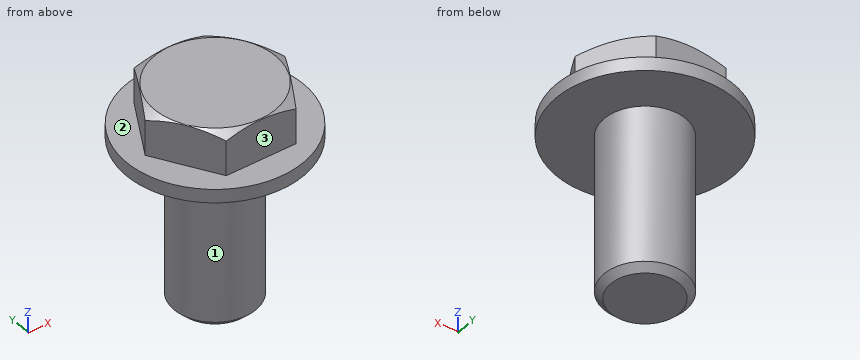
Solid Edge part; units mm, degrees
sketch "Sketch1" plane through (0, 0, 0) normal (0, 0, 1) x (1, 0, 0)
  circle A0 centre (0, 0) radius 6.5
extrude "Protrusion1" add sketch "Sketch1" against normal blind 1
sketch "Sketch2" plane through (0, 0, 0) normal (0, 0, 1) x (1, 0, 0)
  line L0 (2.5981, 4.5) -> (-2.5981, 4.5)
  line L1 (-2.5981, 4.5) -> (-5.1962, 0)
  line L2 (-5.1962, 0) -> (-2.5981, -4.5)
  line L3 (-2.5981, -4.5) -> (2.5981, -4.5)
  line L4 (2.5981, -4.5) -> (5.1962, 0)
  line L5 (5.1962, 0) -> (2.5981, 4.5)
extrude "Protrusion2" add sketch "Sketch2" along normal blind 3
sketch "Sketch3" plane through (0, 0, 0) normal (1, 0, 0) x (0, 1, 0)
  line L0 (-4.45, 3) -> (-7.9141, 1)
revolve "RevolvedCutout1" cut sketch "Sketch3" angle 360 about axis through (0, 0, 2.5) along (0, 0, -1) material side at (0, -6.2071, 2.0433)
sketch "Sketch4" plane through (0, 0, -1) normal (0, 0, -1) x (0, 1, 0)
  circle A0 centre (0, 0) radius 3
extrude "Protrusion3" add sketch "Sketch4" along normal blind 12
chamfer "Chamfer1" distance 0.5 angle 45 1 edges at (0, -3, -13)
properties part number "WHB-6X12" material "STEEL"
Geometry: final body of the model. Coordinates: model frame, mm. Face numbers are marked on the shaded views. A direction names the side the tool comes from. Round coordinates to 2 decimals unless told otherwise and drop trailing zeros. Order: outer loops, then holes, each group sorted by start corner. A loop starts at its lowest first (then second) coordinate and runs counter-clockwise, first axis right, second up.
Q1. Section D-D, the plane z = -6.5. Output: boundary loops of the cut face in (x, y).
Result sheet:
outline: circle Ø6 at (0, 0)
Q2. Pin query (flat end, axial travel): pin 1 (0.9 mm diameter, centred on x = 0.5, z = 2, fed in from -Y); pin 2 (6 mm diameter, centred on x = -0.5, z = -5, fed in from -Y); pin 3 (1.5 mm diameter, centred on x = 1, z = 1, fed in from +Y). Return the tip coordinate at first contact, or that it passes through.
Result sheet:
pin 1: stops at y = -4.5
pin 2: stops at y = -3
pin 3: stops at y = 4.5
Q3. Section A-A, the plane x = 0. Output: boundary loops of the cut face in (y, z), and give its area (3 significant figures).
Result sheet:
outline: (-6.5, -1) - (-3, -1) - (-3, -12.5) - (-2.5, -13) - (2.5, -13) - (3, -12.5) - (3, -1) - (6.5, -1) - (6.5, 0) - (4.5, 0) - (4.5, 2.97) - (4.45, 3) - (-4.45, 3) - (-4.5, 2.97) - (-4.5, 0) - (-6.5, 0) - close
area: 112 mm2
Q4. Access query for the marked faces 1, 2 and 3. Directions: +Z, -Z, +X, -X, +Y, -Y. A direction counts if a zero-diameter tool reaches every point of the face in a straight line with its end or side. Return the directions, or none.
Result sheet:
face 1: -Z
face 2: +Z
face 3: +Z, +X, -X, -Y
Q5. Material intervals for probe 1 along Z at (x, y) = (1, -4.75); probe 2 along Y at (x, z) = (-1.25, 0.5); probe 3 along Z at (x, y) = (0, -4.25), sorted ascending.
Result sheet:
probe 1: z = -1 to 0
probe 2: y = -4.5 to 4.5
probe 3: z = -1 to 3
Q6. Section C-C, the plane y = -4.75. Output: boundary loops of the cut face in (x, z), and give its area (3 significant figures).
Result sheet:
outline: (-4.44, -1) - (4.44, -1) - (4.44, 0) - (-4.44, 0) - close
area: 8.87 mm2
Q7. Section B-B, the plane z = 1.75. Output: boundary loops of the cut face in (x, y), and give its area (3 significant figures).
Result sheet:
outline: (-5.2, 0) - (-2.6, -4.5) - (2.6, -4.5) - (5.2, 0) - (2.6, 4.5) - (-2.6, 4.5) - close
area: 70.1 mm2
